```python
from build123d import *

# Parameters (mm, degrees)
SKETCH_W                      = 32
SKETCH_H                      = 50
PAD_DEPTH                     = 15
SKETCH001_W                   = 27
SKETCH001_H                   = 39
POCKET_DEPTH                  = 13.5
FILLET_R                      = 3
SKETCH002_W                   = 29
SKETCH002_H                   = 47
POCKET001_DEPTH               = 1
FILLET001_R                   = 3
SKETCH003_R                   = 4
POCKET002_DEPTH               = 50.001
SKETCH007_R                   = 1
POCKET004_DEPTH               = 5
SKETCH007_MIRRORED002_2_R     = 1
POCKET004_MIRRORED002_2_DEPTH = 5


with BuildPart() as part:
    # Sketch → Pad (new body)
    with BuildSketch(Plane.XY):
        Rectangle(SKETCH_W, SKETCH_H)
    extrude(amount=PAD_DEPTH)

    # Sketch001 (on Face6 of Pad) → Pocket (cut)
    with BuildSketch(Plane.XY.offset(15)):
        Rectangle(SKETCH001_W, SKETCH001_H)
    extrude(amount=-POCKET_DEPTH, mode=Mode.SUBTRACT)

    # Fillet
    fillet_edges = [part.edges().sort_by_distance(p)[0] for p in [
        (-16, -25, 7.5),
        (16, -25, 7.5),
        (-16, 25, 7.5),
        (16, 25, 7.5),
    ]]
    fillet(fillet_edges, radius=FILLET_R)

    # Sketch002 (on Face5 of Fillet) → Pocket001 (cut)
    with BuildSketch(Plane.XY.offset(15)):
        Rectangle(SKETCH002_W, SKETCH002_H)
    extrude(amount=-POCKET001_DEPTH, mode=Mode.SUBTRACT)

    # Fillet001
    fillet001_edges = [part.edges().sort_by_distance(p)[0] for p in [
        (-14.5, 23.5, 14.5),
        (14.5, 23.5, 14.5),
        (-14.5, -23.5, 14.5),
        (14.5, -23.5, 14.5),
    ]]
    fillet(fillet001_edges, radius=FILLET001_R)

    # Sketch003 (on Face17 of Fillet001) → Pocket002 (cut, through all)
    with BuildSketch(Plane.XZ.offset(25)):
        with Locations((0, 7.5)):
            Circle(SKETCH003_R)
    extrude(amount=-POCKET002_DEPTH, mode=Mode.SUBTRACT)

    # Sketch007 (on Face18 of Pocket002) → Pocket004 (cut)
    with BuildSketch(Plane.XY.offset(14)):
        with Locations((-11.5, 21.5)):
            Circle(SKETCH007_R)
    pocket004 = extrude(amount=-POCKET004_DEPTH, mode=Mode.SUBTRACT)

    # Sketch007 Mirrored002 2 → Pocket004 Mirrored002 2 (cut)
    with BuildSketch(Plane(origin=(0, 0, 14), x_dir=(-1, 0, 0), z_dir=(0, 0, -1))):
        with Locations((-11.5, 21.5)):
            Circle(SKETCH007_MIRRORED002_2_R)
    pocket004_mirrored002_2 = extrude(amount=POCKET004_MIRRORED002_2_DEPTH, mode=Mode.SUBTRACT)

    # Mirrored003: Pocket004, Pocket004 Mirrored002 2 across Sketch007 H_Axis
    add(pocket004.mirror(Plane(origin=(0, 0, 14), x_dir=(0, 0, 1), z_dir=(0, 1, 0))), mode=Mode.SUBTRACT)
    add(pocket004_mirrored002_2.mirror(Plane(origin=(0, 0, 14), x_dir=(0, 0, 1), z_dir=(0, 1, 0))), mode=Mode.SUBTRACT)


solid = part.part
```
Build history of the part. All positions in model axes, mm. A direction names the side the tool comes from. Coordinates: 2 decimals unless noted, no trailing zeros. Order: outer loops, then holes, each group sorted by start corner. A loop starts at its lowest first (then second) coordinate and runs counter-clockwise, first axis right, second up.
Item 1: Drop flat-ended pins along their axis: pin 1 Ø6 at (x, z) = (2.5, 6.5) entering from +Y; pin 2 Ø1.5 at (x, y) = (-6.5, -5.5) entering from +Z; pin 3 Ø1 at (x, y) = (-12, 22) entering from +Z; pin 4 Ø1 at (x, y) = (-11.5, -21.5) entering from +Z. Give the stop position or say it passes through.
Filled in:
pin 1: stops at y = 25
pin 2: stops at z = 1.5
pin 3: stops at z = 14
pin 4: stops at z = 9
Item 2: Drill centre lines: L1, parallel to Y at x = 11.5, z = 12.05; L2, parallel to Y at x = -7, z = 1.75; L3, parallel to Z at x = 0, y = 21. Where is each one in solid material? Low to high.
Filled in:
L1: y = -25 to -22.5, -20.5 to -19.5, 19.5 to 20.5, 22.5 to 25
L2: y = -25 to -19.5, 19.5 to 25
L3: z = 0 to 3.5, 11.5 to 14
Item 3: Saw through at A-A on x = 0. List the corners of the cut face in (y, z).
Filled in:
outline: (-25, 0) - (25, 0) - (25, 3.5) - (19.5, 3.5) - (19.5, 1.5) - (-19.5, 1.5) - (-19.5, 3.5) - (-25, 3.5) - close; (-25, 11.5) - (-19.5, 11.5) - (-19.5, 14) - (-23.5, 14) - (-23.5, 15) - (-25, 15) - close; (19.5, 11.5) - (25, 11.5) - (25, 15) - (23.5, 15) - (23.5, 14) - (19.5, 14) - close
Item 4: Tool access for faces 5 (the cylindrical face through (13.64, 22.6, 14.49)), 6 (the flat face through (0, 0, 0)): list every direction of +Z, -Z, +X, -X, +Y, -Y with a clear straight run to the whole face (end or side of a thin tool).
Filled in:
face 5: +Z
face 6: -Z, +X, -X, +Y, -Y
Item 5: Saw through at C-C on z = 12.5. List the corners of the cut face in (x, y), then the cut area to 3 significant figures.
Filled in:
outline: (-16, -22) arc R3 ccw to (-13, -25) - (13, -25) arc R3 ccw to (16, -22) - (16, 22) arc R3 ccw to (13, 25) - (-13, 25) arc R3 ccw to (-16, 22) - close; hole (-13.5, -19.5) - (13.5, -19.5) - (13.5, 19.5) - (-13.5, 19.5) - close; hole circle Ø2 at (-11.5, -21.5); hole circle Ø2 at (-11.5, 21.5); hole circle Ø2 at (11.5, -21.5); hole circle Ø2 at (11.5, 21.5)
area: 527 mm2
Item 6: Mould opens along Y. For faces 1 (the flat face through (-15, 0, 15)), 2 (the flat face through (-12, -22, 9)), 3 (the flat face through (-3, -25, 4)), 4 (the cylindrical face through (15.1, 24.14, 7.6)) say: released by +Y, released by -Y, zero draft, split by the parting line, or undercut.
Filled in:
face 1: zero draft
face 2: undercut
face 3: released by -Y
face 4: released by +Y
Item 7: Saw through at B-B on z = 7.5. List the corners of the cut face in (x, y).
Filled in:
outline: (-16, -22) arc R3 ccw to (-13, -25) - (-4, -25) - (-4, -19.5) - (-13.5, -19.5) - (-13.5, 19.5) - (-4, 19.5) - (-4, 25) - (-13, 25) arc R3 ccw to (-16, 22) - close; (4, -25) - (13, -25) arc R3 ccw to (16, -22) - (16, 22) arc R3 ccw to (13, 25) - (4, 25) - (4, 19.5) - (13.5, 19.5) - (13.5, -19.5) - (4, -19.5) - close
Item 8: Saw through at D-D on y = 14.5. List the corners of the cut face in (x, z).
Filled in:
outline: (-16, 0) - (16, 0) - (16, 15) - (14.5, 15) - (14.5, 14) - (13.5, 14) - (13.5, 1.5) - (-13.5, 1.5) - (-13.5, 14) - (-14.5, 14) - (-14.5, 15) - (-16, 15) - close
